from build123d import *

# Parameters (mm, degrees)
SKETCH_1_R          = 1.4
SKETCH_1_W          = 3
SKETCH_1_H          = 12
EXTRUDE_1_DEPTH     = 3
SKETCH_2_W          = 20
SKETCH_2_H          = 3
EXTRUDE_2_DEPTH     = 2.8
SKETCH_3_W          = 3
SKETCH_3_H          = 12
EXTRUDE_3_DEPTH     = 3
SKETCH_4_W          = 3
SKETCH_4_H          = 3.946305982
CUT_EXTRUDE_1_DEPTH = 3
SKETCH_5_W          = 3
SKETCH_5_H          = 3
CUT_EXTRUDE_2_DEPTH = 1
SKETCH_7_W          = 3
SKETCH_7_H          = 2.8
CUT_EXTRUDE_4_DEPTH = 60
CUT_EXTRUDE_5_DEPTH = 60
EXTRUDE_4_DEPTH     = 3
FILLET_1_R          = 3
EXTRUDE_START       = -3
EXTRUDE_5_DEPTH     = 3
CUT_EXTRUDE_7_DEPTH = 10


with BuildPart() as part:
    # 草图1 → 凸台-拉伸1 (new body)
    with BuildSketch(Plane.XY):
        Polygon((-54.8, 15.675), (-67.8, 15.675), (-70.8, 12.675), (-70.8, -11.325), (-67.8, -14.325), (-49.8, -14.325), (-49.8, -17.325), (-39.8, -17.325), (-39.8, -14.325), (-22, -14.325), (-22, -2.975), (-17, -2.970818371), (-17, -14.325), (-10, -14.325), (-10, -17.325), (10, -17.325), (10, -14.325), (17, -14.325), (17, -2.970818371), (22, -2.975), (22, -14.325), (39.8, -14.325), (39.8, -17.325), (49.8, -17.325), (49.8, -14.325), (67.8, -14.325), (70.8, -11.325), (70.8, 12.675), (67.8, 15.675), (54.8, 15.675), (54.8, 12.875), (29.8, 12.875), (29.8, 15.675), (10, 15.675), (10, 12.875), (-10, 12.875), (-10, 15.675), (-29.8, 15.675), (-29.8, 12.875), (-54.8, 12.875), align=None)
        with Locations((-62.3, 9.063133886)):
            Circle(SKETCH_1_R, mode=Mode.SUBTRACT)
        with Locations((62.3, 9.063133886)):
            Circle(SKETCH_1_R, mode=Mode.SUBTRACT)
        with Locations((-63.3, -0.325)):
            Rectangle(SKETCH_1_W, SKETCH_1_H, mode=Mode.SUBTRACT)
        with Locations((63.3, -0.325)):
            Rectangle(SKETCH_1_W, SKETCH_1_H, mode=Mode.SUBTRACT)
    extrude(amount=EXTRUDE_1_DEPTH)

    # 草图2 → 凸台-拉伸2 (add)
    with BuildSketch(Plane(origin=(0, 12.875, 0), x_dir=(1, 0, 0), z_dir=(0, 1, 0))):
        with Locations((0, -1.5)):
            Rectangle(SKETCH_2_W, SKETCH_2_H)
    extrude(amount=EXTRUDE_2_DEPTH)

    # 草图3 → 凸台-拉伸3 (add)
    with BuildSketch(Plane.XY.offset(3)):
        with Locations((-63.3, -0.325)):
            Rectangle(SKETCH_3_W, SKETCH_3_H)
        with Locations((63.3, -0.325)):
            Rectangle(SKETCH_3_W, SKETCH_3_H)
    extrude(amount=-EXTRUDE_3_DEPTH)

    # 草图4 → 切除-拉伸1 (cut)
    with BuildSketch(Plane(origin=(133.943153128, -125.945742166, 0), x_dir=(1, 0, 0), z_dir=(0, 0, -1))):
        Polygon((-72.143153128, -111.674436184), (-72.143153128, -127.209199434), (-69.143153128, -127.209199434), (-69.143153128, -111.674436184), (-69.143153128, -111.620742166), (-72.143153128, -111.620742166), align=None)
        with Locations((-70.643153128, -109.647589175)):
            Rectangle(SKETCH_4_W, SKETCH_4_H)
    cut_extrude_1 = extrude(amount=-CUT_EXTRUDE_1_DEPTH, mode=Mode.SUBTRACT)

    # 镜向1: 切除-拉伸1 across plane
    add(cut_extrude_1.mirror(Plane.ZY), mode=Mode.SUBTRACT)

    # 草图5 → 切除-拉伸2 (cut)
    with BuildSketch(Plane.XZ.offset(-1.263457268)):
        with Locations((63.3, 1.5)):
            Rectangle(SKETCH_5_W, SKETCH_5_H)
        with Locations((-63.3, 1.5)):
            Rectangle(SKETCH_5_W, SKETCH_5_H)
    extrude(amount=-CUT_EXTRUDE_2_DEPTH, mode=Mode.SUBTRACT)

    # 草图7 → 切除-拉伸4 (cut)
    with BuildSketch(Plane(origin=(29.8, 0, 0), x_dir=(0, 0, -1), z_dir=(1, 0, 0))):
        with Locations((-1.5, 14.275)):
            Rectangle(SKETCH_7_W, SKETCH_7_H)
    extrude(amount=-CUT_EXTRUDE_4_DEPTH, mode=Mode.SUBTRACT)

    # 草图8 → 切除-拉伸5 (cut)
    with BuildSketch(Plane(origin=(0, 0, 0), x_dir=(-1, 0, 0), z_dir=(0, 0, -1))):
        Polygon((-8, 0), (-13, 0), (-22, 12.875), (-17, 12.875), (17, 12.875), (22, 12.875), (13, 0), (8, 0), (0, 0), align=None)
    extrude(amount=-CUT_EXTRUDE_5_DEPTH, mode=Mode.SUBTRACT)

    # 草图10 → 凸台-拉伸4 (add)
    with BuildSketch(Plane(origin=(0, 0, 0), x_dir=(-1, 0, 0), z_dir=(0, 0, -1))):
        Polygon((-22, 12.875), (-13, 0), (13, 0), (22, 12.875), (19.559801877, 12.875), (11.95786013, 2), (-11.95786013, 2), (-19.559801877, 12.875), align=None)
    extrude(amount=-EXTRUDE_4_DEPTH)

    # 圆角1
    fillet_1_edges = [part.edges().sort_by_distance(p)[0] for p in [
        (-11.95786013, 2, 1.5),
        (11.95786013, 2, 1.5),
    ]]
    fillet(fillet_1_edges, radius=FILLET_1_R)

    # 草图11 → 凸台-拉伸5 (add)
    with BuildSketch(Plane(origin=(0, 0, 0), x_dir=(-1, 0, 0), z_dir=(0, 0, -1)).offset(EXTRUDE_START)):
        with BuildLine():
            Line((-12.853467068, 3.281215481), (-19.559801877, 12.875))
            Line((-19.559801877, 12.875), (-18.339702816, 12.875))
            Line((-18.339702816, 12.875), (-12.033861487, 3.854143654))
            ThreePointArc((-12.033861487, 3.854143654), (-11.31884925, 3.226343791), (-10.394650325, 3))
            Line((-10.394650325, 3), (10.394650325, 3))
            ThreePointArc((10.394650325, 3), (11.31884925, 3.226343791), (12.033861487, 3.854143654))
            Line((12.033861487, 3.854143654), (18.339702816, 12.875))
            Line((18.339702816, 12.875), (19.559801877, 12.875))
            Line((19.559801877, 12.875), (12.853467068, 3.281215481))
            ThreePointArc((12.853467068, 3.281215481), (11.780948713, 2.339515687), (10.394650325, 2))
            Line((10.394650325, 2), (-10.394650325, 2))
            ThreePointArc((-10.394650325, 2), (-11.780948713, 2.339515687), (-12.853467068, 3.281215481))
        make_face()
    extrude(amount=EXTRUDE_5_DEPTH)

    # 草图12 → 切除-拉伸7 (cut)
    with BuildSketch(Plane(origin=(0, 0, 0), x_dir=(-1, 0, 0), z_dir=(0, 0, -1))):
        Polygon((-22, -2.975), (-22, -14.325), (-22.05, -14.325), (-22.05, -2.925041799), (-16.95, -2.920776537), (-16.95, -14.325), (-17, -14.325), (-17, -2.970818371), align=None)
        Polygon((17, -2.970818371), (17, -14.325), (16.95, -14.325), (16.95, -2.920776537), (22.05, -2.925041799), (22.05, -14.325), (22, -14.325), (22, -2.975), align=None)
    extrude(amount=-CUT_EXTRUDE_7_DEPTH, mode=Mode.SUBTRACT)


solid = part.part
Source: CAD feature listing. Evaluate the final solid. Frame: model axes, mm. A direction names the side the tool comes from. Give positions to 0.01 mm unless a question says otherwise; leave off trailing zeros. Write each loop counter-clockwise with the first axis right and the second up, starting at its lowest first coordinate (ties: lowest second). Pieces come first, ordered by that corner, then holes. Notation, with made-up numbers: (63.5, 17.5) - (112.5, 17.5) arc R28 cw to (112.5, 49.5) - close; hole circle Ø11 at (23.25, 51.25). An arc over 180 degrees is marked (long way). Write item = value, one per line. Start each with the question number.
Q1. Cut plane D-D, the plane x = 14.5. Return loops of the section in (y, z) (3 decimals), then the cut area to 3 significant figures.
Q2. Pin query (flat end, axial travel): pin 1 Ø0.9 at (x, z) = (14.5, 1.5) entering from -Y (3 decimals); pin 2 Ø0.9 at (x, z) = (62.5, 2) entering from -Y; pin 3 Ø1.5 at (x, z) = (41, 1) entering from +Y (3 decimals). Return the tip coordinate at first contact, or that it passes through.
Q3. Cut plane B-B, the plane x = 46.5. Return loops of the section in (y, z) (3 decimals), then the cut area to 3 significant figures.
Q4. Material intervals for probe 1 along X at (y, z) = (-11, 2.15); probe 2 along X at (y, z) = (-1, 2); probe 3 along Y at (x, z) = (62.3, 2.1) (3 decimals), sorted ascending.
Q5. Draft query along Y for faces 1 (the flat face through (15.231, 8.428, 1.521)), 2 (the flat face through (31, -14.325, 1)), 3 (the flat face through (-22.05, -9, 1)), 4 (the cylindrical face through (60.9, 9.1, 1.5)). Return one class per face: +Y half, -Y half, draft (parallel to the pull), parting line (faces both ways), or undercut.
Q6. Cut plane A-A, the plane y = -10. Return loops of the section in (x, z), then the cut area to 3 significant figures.
Q7. Cut plane C-C, the plane z = 1.1. Give the number of separate pieces and of enclosed holes in the cut face, then the cut area to 3 significant figures.
Q8. Reachability of faces 5 (the flat face through (61, 15.675, 1)), 6 (the flat face through (64.8, -6, 1)), 7 (the flat face through (-54.8, 14, 1)) from +Z, -Z, +X, -X, +Y, -Y: full face, straight path, thin tool, end or side. Return the list, or none.
Computed values:
q1.outline = (-14.325, 0) - (7.382, 0) - (7.382, 3) - (-14.325, 3) - close
q1.area = 65.1 mm²
q2.pin_1 = -14.325
q2.pin_2 = 2.26
q2.pin_3 = 12.875
q3.outline = (-17.325, 0) - (12.875, 0) - (12.875, 3) - (-17.325, 3) - close
q3.area = 90.6 mm²
q4.probe_1 = -70.8 to -64.8, -61.8 to -22.05, -16.95 to 16.95, 22.05 to 61.8, 64.8 to 70.8
q4.probe_2 = -70.8 to -64.8, -61.8 to 61.8, 64.8 to 70.8
q4.probe_3 = 2.263 to 7.663, 10.463 to 15.675
q5.face_1 = +Y half
q5.face_2 = -Y half
q5.face_3 = draft
q5.face_4 = undercut
q6.outline = (-70.8, 0) - (-64.8, 0) - (-64.8, 3) - (-70.8, 3) - close; (-61.8, 0) - (-22.05, 0) - (-22.05, 3) - (-61.8, 3) - close; (-16.95, 0) - (16.95, 0) - (16.95, 3) - (-16.95, 3) - close; (22.05, 0) - (61.8, 0) - (61.8, 3) - (22.05, 3) - close; (64.8, 0) - (70.8, 0) - (70.8, 3) - (64.8, 3) - close
q6.area = 376 mm²
q7.separate_pieces = 1
q7.enclosed_holes = 2
q7.area = 3,520 mm²
q8.face_5 = +Z, -Z, +X, -X, +Y
q8.face_6 = +Z, -Z, -Y
q8.face_7 = +Z, -Z, +Y
